Geometry check sheet. Reference: the model listing, model coordinates, mm. A direction names the side the tool comes from. Coordinates: 2 decimals unless noted, no trailing zeros. Loops run counter-clockwise (first coordinate to the right, second up) from the corner with the lowest first, then second, coordinate; pieces in that order, holes last.
from build123d import *

# Parameters (mm, degrees)
CROQUIS1_R              = 5
SALIENTE_EXTRUIR1_DEPTH = 10
CROQUIS2_R              = 33
SALIENTE_EXTRUIR2_DEPTH = 15
CROQUIS3_R              = 1.5


with BuildPart() as part:
    # Croquis1 → Saliente-Extruir1 (new body)
    with BuildSketch(Plane.XY):
        Circle(CROQUIS1_R)
        with BuildLine():
            Line((-2.236067977, -2), (2.236067977, -2))
            ThreePointArc((2.236067977, -2), (3, 0), (2.236067977, 2))
            Line((2.236067977, 2), (-2.236067977, 2))
            ThreePointArc((-2.236067977, 2), (-3, 0), (-2.236067977, -2))
        make_face(mode=Mode.SUBTRACT)
    extrude(amount=SALIENTE_EXTRUIR1_DEPTH)

    # Croquis2 → Saliente-Extruir2 (add)
    with BuildSketch(Plane.XY.offset(10)):
        Circle(CROQUIS2_R)
    extrude(amount=SALIENTE_EXTRUIR2_DEPTH)

    # Croquis3 → Cortar-Revolución1 (revolve, cut)
    with BuildSketch(Plane(origin=(0, 0, 0), x_dir=(1, 0, 0), z_dir=(0, 1, 0))):
        with Locations((33, -15)):
            Circle(CROQUIS3_R)
        with Locations((33, -20)):
            Circle(CROQUIS3_R)
    revolve(axis=Axis((0, 0, 24.978866337), (0, 0, -1)), mode=Mode.SUBTRACT)


solid = part.part
1) Section check C-C on y = 0. Record the cut outline in (x, z), and give its area (3 significant figures).
Data:
outline: (-33, 10) - (-5, 10) - (-5, 0) - (-3, 0) - (-3, 10) - (3, 10) - (3, 0) - (5, 0) - (5, 10) - (33, 10) - (33, 13.5) arc R1.5 cw to (33, 16.5) - (33, 18.5) arc R1.5 cw to (33, 21.5) - (33, 25) - (-33, 25) - (-33, 21.5) arc R1.5 cw to (-33, 18.5) - (-33, 16.5) arc R1.5 cw to (-33, 13.5) - close
area: 1,020 mm2
2) Depth check by flat-ended pin: pin 1 (12 mm diameter, centred on x = -14.5, y = -6.5, fed in from -Z); pin 2 (1.5 mm diameter, centred on y = -12.5, z = 19, fed in from +X); pin 3 (8 mm diameter, centred on x = 20, z = 8.5, fed in from -Y). Enter the tip coordinate at first touch or a pass-through.
Data:
pin 1: stops at z = 10
pin 2: stops at x = 30.76
pin 3: stops at y = -28.7
3) Access from +Z, -Z, +X, -X, +Y, -Y to the whole of each face (thin tool, end or side, straight path). Record for faces 4 (the flat face through (0, 0, 10)), 5 (the cylindrical face through (30.5, -12.6, 23.2)).
Data:
face 4: -Z
face 5: +Z, -Z
4) Material ranges on probe 1 along Z at (x, y) = (-15, 29); probe 2 along Z at (x, y) = (14.5, 24.5); probe 3 along Y at (x, z) = (-4, 9.5), recorded low to high.
Data:
probe 1: z = 10 to 13.54, 16.46 to 18.54, 21.46 to 25
probe 2: z = 10 to 25
probe 3: y = -3 to 3
5) Section check A-A on x = 0. Record the cut outline in (y, z), and give its area (3 significant figures).
Data:
outline: (-33, 10) - (-5, 10) - (-5, 0) - (-2, 0) - (-2, 10) - (2, 10) - (2, 0) - (5, 0) - (5, 10) - (33, 10) - (33, 13.5) arc R1.5 cw to (33, 16.5) - (33, 18.5) arc R1.5 cw to (33, 21.5) - (33, 25) - (-33, 25) - (-33, 21.5) arc R1.5 cw to (-33, 18.5) - (-33, 16.5) arc R1.5 cw to (-33, 13.5) - close
area: 1,040 mm2
6) Section check B-B on z = 7.25. Record the cut outline in (x, y), and give its area (3 significant figures).
Data:
outline: circle Ø10 at (0, 0); hole (-2.24, -2) - (2.24, -2) arc R3 ccw to (2.24, 2) - (-2.24, 2) arc R3 ccw to start
area: 56.5 mm2
7) Mould release check, pull along Y, two halves, no side actions. Record for faces 1 (the cylindrical face through (30.5, -12.6, 17.5)), 2 (the flat face through (0, 2, 5)), 3 (the flat face through (0, 0, 25)): +Y half, -Y half, draft (parallel to the pull), parting line (faces both ways), or undercut.
Data:
face 1: parting line
face 2: undercut
face 3: draft
